Build history of the part. All positions in model axes, mm. A direction names the side the tool comes from. Round coordinates to 2 decimals unless told otherwise and drop trailing zeros. Write each loop counter-clockwise with the first axis right and the second up, starting at its lowest first coordinate (ties: lowest second). Pieces come first, ordered by that corner, then holes.
Item 1: Mould opens along Y. For faces 3 (the flat face through (-7, 500, 99)), 4 (the flat face through (-7, -500, 99)), 5 (the flat face through (-500, -7, 99)), 6 (the flat face through (-200, 150, 175)) say: +Y half, -Y half, draft (parallel to the pull), parting line (faces both ways), or undercut.
Item 2: Band-saw the part on B-B, the plane z = 181. Write the cut outline in (x, y), then the cut area to 3 significant figures.
Item 3: Wall check: probe 1 along X at (y, z) = (-164, 168.5); probe 2 along Y at (x, z) = (138.5, 163.5); probe 3 along X at (y, z) = (-47.5, 155). Give the ranges that are in metal, low to high.
Item 4: Band-saw the part on A-A, the plane x = -250.5. Write the cut outline in (y, z).
Item 5: 3-axis set-ups, long thin cutter, end or side, ignore diameter. For faces 1 (the flat face through (-300, 4, 175)), 2 (the flat face through (-7, 7, 0)): which of +Z, -Z, +X, -X, +Y, -Y reach the whole face in a straight line?
Item 6: Band-saw the part on C-C, the plane y = 209. Write the cut outline in (x, z), then the cut area to 3 significant figures.
Item 7: Drop a flat-ended pin along its axis: pin 1 Ø2 at (x, y) = (8, -35.5) entering from +Z. Give the stop position or say it passes through.
```python
from build123d import *

# Parameters (mm, degrees)
SKETCH_W     = 1000
SKETCH_H     = 1000
PAD_DEPTH    = 200
POCKET_DEPTH = 50


with BuildPart() as part:
    # Sketch → Pad (new body)
    with BuildSketch(Plane.XY):
        Rectangle(SKETCH_W, SKETCH_H)
    extrude(amount=PAD_DEPTH)

    # Sketch001 → Pocket (cut)
    with BuildSketch(Plane.XY.offset(200)):
        Polygon((-300, 253.105738), (-300, -253.105738), (-200, -253.105738), (-200, -50), (300, -50), (300, 50), (-200, 50), (-200, 253.105738), align=None)
    extrude(amount=-POCKET_DEPTH, mode=Mode.SUBTRACT)


solid = part.part
```
Results:
1. face 3: +Y half
1. face 4: -Y half
1. face 5: draft
1. face 6: undercut
2. outline: (-500, -500) - (500, -500) - (500, 500) - (-500, 500) - close; hole (-300, -253.11) - (-200, -253.11) - (-200, -50) - (300, -50) - (300, 50) - (-200, 50) - (-200, 253.11) - (-300, 253.11) - close
2. area: 899,000 mm2
3. probe 1: x = -500 to -300, -200 to 500
3. probe 2: y = -500 to -50, 50 to 500
3. probe 3: x = -500 to -300, 300 to 500
4. outline: (-500, 0) - (500, 0) - (500, 200) - (253.11, 200) - (253.11, 150) - (-253.11, 150) - (-253.11, 200) - (-500, 200) - close
5. face 1: +Z
5. face 2: -Z, +X, -X, +Y, -Y
6. outline: (-500, 0) - (500, 0) - (500, 200) - (-200, 200) - (-200, 150) - (-300, 150) - (-300, 200) - (-500, 200) - close
6. area: 195,000 mm2
7. pin 1: stops at z = 150
